from build123d import *

# Parameters (mm, degrees)
SKETCH2_R           = 10.5
BOSS_EXTRUDE1_DEPTH = 25
SKETCH3_W           = 21
SKETCH3_H           = 21
BOSS_EXTRUDE2_DEPTH = 50
SKETCH4_R           = 10.5
BOSS_EXTRUDE3_DEPTH = 25
SKETCH5_W           = 10
SKETCH5_H           = 10
BOSS_EXTRUDE4_DEPTH = 10
SKETCH6_R           = 4
CUT_EXTRUDE1_DEPTH  = 18
SKETCH7_R           = 6.5
CUT_EXTRUDE2_DEPTH  = 65


with BuildPart() as part:
    # Sketch2 → Boss-Extrude1 (new body)
    with BuildSketch(Plane(origin=(0, 0, 0), x_dir=(1, 0, 0), z_dir=(0, 1, 0))):
        with Locations(Location((0, 0, 0), (0, 0, 270))):
            Circle(SKETCH2_R)
    extrude(amount=BOSS_EXTRUDE1_DEPTH)

    # Sketch3 → Boss-Extrude2 (add)
    with BuildSketch(Plane(origin=(0, 25, 0), x_dir=(1, 0, 0), z_dir=(0, 1, 0))):
        Rectangle(SKETCH3_W, SKETCH3_H)
    extrude(amount=BOSS_EXTRUDE2_DEPTH)

    # Sketch4 → Boss-Extrude3 (add)
    with BuildSketch(Plane(origin=(0, 75, 0), x_dir=(1, 0, 0), z_dir=(0, 1, 0))):
        with Locations(Location((0, 0, 0), (0, 0, 270))):
            Circle(SKETCH4_R)
    extrude(amount=BOSS_EXTRUDE3_DEPTH)

    # Sketch5 → Boss-Extrude4 (add)
    with BuildSketch(Plane(origin=(0, 100, 0), x_dir=(1, 0, 0), z_dir=(0, 1, 0))):
        Rectangle(SKETCH5_W, SKETCH5_H)
    extrude(amount=BOSS_EXTRUDE4_DEPTH)

    # Sketch6 → Cut-Extrude1 (cut)
    with BuildSketch(Plane.ZY.offset(10.5)):
        with Locations((0, 56.203092856)):
            Circle(SKETCH6_R)
    extrude(amount=-CUT_EXTRUDE1_DEPTH, mode=Mode.SUBTRACT)

    # Sketch7 → Cut-Extrude2 (cut)
    with BuildSketch(Plane.XZ):
        with Locations(Location((0, 0, 0), (0, 0, 270))):
            Circle(SKETCH7_R)
    extrude(amount=-CUT_EXTRUDE2_DEPTH, mode=Mode.SUBTRACT)


solid = part.part
Here's how the part is built. I have some questions about the finished solid (model axes, mm). A direction names the side the tool comes from. Coordinates: 2 decimals unless noted, no trailing zeros. Write each loop counter-clockwise with the first axis right and the second up, starting at its lowest first coordinate (ties: lowest second). Pieces come first, ordered by that corner, then holes.
Item 1: If we mould it in two halves opening along Z, with no side actions, what happens to faces 6 (the cylindrical face through (6.445, 32.045, 0.846)), 7 (the flat face through (-8, 75, 8)), 8 (the flat face through (0, 50, 10.5))? For each: +Z half, -Z half, draft (parallel to the pull), parting line (faces both ways), or undercut.
Item 2: I want a section at C-C on x = -8.5. Write out the boundary of the cut face in (y, z).
Item 3: I want a section at D-D on x = 2. Write out the boundary of the cut face in (y, z), and give its area (3 significant figures).
Item 4: Will these pins go through, and if not, where does the flat tip stop? pin 1 (10.5 mm diameter, centred on x = 0, z = 0, fed in from -Y); pin 2 (1.5 mm diameter, centred on x = -2.5, y = 96, fed in from -Z); pin 3 (5 mm diameter, centred on x = -1.5, y = 103, fed in from +Z).
Item 5: If I drill on line 1 (X direction, y = 17, z = 0); line 2 (Z direction, x = 0.5, y = 40.5); line 3 (Y direction, x = 5.8, z = 0), over which ranges is the centre line in solid material (lowest first)?
Item 6: I want a section at B-B on y = 50.5. Write out the boundary of the cut face in (x, z), and give its area (3 significant figures).
Item 7: I want a section at A-A on z = -1.75. Write out the boundary of the cut face in (x, y).
Item 8: On a 3-axis mill with a long thin cutter (end or side, diameter ignored), from which of +Z, -Z, +X, -X, +Y, -Y can I reach the whole of each face in a straight line? I mean faces 1 (the flat face through (5, 105, 0)), 2 (the flat face through (0, 105, -5)), 3 (the flat face through (-8, 25, -8)), 4 (the flat face through (8, 25, -8)), 5 (the cylindrical face through (-8.447, 54.671, 3.695)). Say none if no direction works.
Findings below:
1. face 6: undercut
1. face 7: draft
1. face 8: +Z half
2. outline: (0, -6.16) - (25, -6.16) - (25, -10.5) - (75, -10.5) - (75, -6.16) - (100, -6.16) - (100, 6.16) - (75, 6.16) - (75, 10.5) - (25, 10.5) - (25, 6.16) - (0, 6.16) - close; hole circle Ø8 at (56.2, 0)
3. outline: (0, -10.31) - (25, -10.31) - (25, -10.5) - (75, -10.5) - (75, -10.31) - (100, -10.31) - (100, -5) - (110, -5) - (110, 5) - (100, 5) - (100, 10.31) - (75, 10.31) - (75, 10.5) - (25, 10.5) - (25, 10.31) - (0, 10.31) - (0, 6.18) - (65, 6.18) - (65, -6.18) - (0, -6.18) - close
3. area: 1,380 mm2
4. pin 1: stops at y = 65
4. pin 2: stops at z = -10.35
4. pin 3: stops at z = 5
5. line 1: x = -10.5 to -6.5, 6.5 to 10.5
5. line 2: z = -10.5 to -6.48, 6.48 to 10.5
5. line 3: y = 65 to 100
6. outline: (-10.5, -10.5) - (10.5, -10.5) - (10.5, 10.5) - (-10.5, 10.5) - close; hole circle Ø13 at (0, 0)
6. area: 308 mm2
7. outline: (-10.5, 25) - (-10.35, 25) - (-10.35, 0) - (-6.26, 0) - (-6.26, 52.61) - (-10.5, 52.61) - close; (-10.5, 59.8) - (-6.26, 59.8) - (-6.26, 65) - (6.26, 65) - (6.26, 59.8) - (7.5, 59.8) - (7.5, 52.61) - (6.26, 52.61) - (6.26, 0) - (10.35, 0) - (10.35, 25) - (10.5, 25) - (10.5, 75) - (10.35, 75) - (10.35, 100) - (5, 100) - (5, 110) - (-5, 110) - (-5, 100) - (-10.35, 100) - (-10.35, 75) - (-10.5, 75) - close
8. face 1: +Z, -Z, +X, +Y
8. face 2: -Z, +X, -X, +Y
8. face 3: -Z, -X, -Y
8. face 4: -Z, +X, -Y
8. face 5: -X
